Verification items for the finished model (mm, model axes). A direction names the side the tool comes from. Coordinates: 2 decimals unless noted, no trailing zeros. Order: outer loops, then holes, each group sorted by start corner. A loop starts at its lowest first (then second) coordinate and runs counter-clockwise, first axis right, second up. Notation, with made-up numbers: (10, 19.5) -> (47, 19.5) arc R24 ccw to (47, 39.5) -> close; hole circle Ø9 at (-11.75, 36). An arc over 180 degrees is marked (long way). Use CSV: the item, a comma, the result in double quotes. Start each with the question number.
1) Sectioned sample at A-A on z = -16. Record the boundary of the cut face in (x, y), then the cut area to 3 significant figures.
2) Go/stop test with flat-tipped pins: pin 1 (5 mm diameter, centred on x = 16, y = 8.5, fed in from -Z); pin 2 (5 mm diameter, centred on x = 5, z = -25, fed in from -Y); pin 3 (1.5 mm diameter, centred on y = 2, z = -17, fed in from +X); pin 4 (1 mm diameter, centred on x = 24, y = 8, fed in from +Z). Record where each tip stops, or that it passes through.
3) Sectioned sample at D-D on z = 0. Record the boundary of the cut face in (x, y).
4) Scan lines: line 1 along X through (y, z) = (2, -25); line 2 along Y through (x, z) = (0, -34); line 3 along X through (y, z) = (2, -26.5). Record each from-to range of solid material in increasing order.
5) Sectioned sample at C-C on x = 24.5. Record the boundary of the cut face in (y, z).
6) Tool access check on faces 4 (the cylindrical face through (4, 7.9, -53.7)), 5 (the flat face through (1.478, 7.93, -33.488)), 6 (the flat face through (12.5, 1, -16)). Record the directions out of +Z, -Z, +X, -X, +Y, -Y that give a thin tool (end or side, any length) a straight path to the whole face; none if there is none.
7) Release check for a two-part mould opening along Z. For faces 1 (the cylindrical face through (-7.186, 14.479, -39.317)), 2 (the cylindrical face through (12.186, 1.521, -5.276)), 3 (the flat face through (19.036, 7.888, -38.273)) record: released by +Z, released by -Z, zero draft, split by the parting line, or undercut.
8) Sectioned sample at B-B on y = 10.5. Record the boundary of the cut face in (x, z), then the cut area to 3 significant figures.
from build123d import *

# Parameters (mm, degrees)
SKETCH1_R           = 2
BOSS_EXTRUDE1_DEPTH = 3
FILLET1_R           = 10
BOSS_EXTRUDE2_DEPTH = 10
BOSS_EXTRUDE3_START = 10
SKETCH2_3_R         = 2
BOSS_EXTRUDE3_DEPTH = 3
CUT_EXTRUDE1_DEPTH  = 74.447466489


with BuildPart() as part:
    # Sketch1 → Boss-Extrude1 (new body)
    with BuildSketch(Plane(origin=(0, 0, 0), x_dir=(1, 0, 0), z_dir=(0, 1, 0))):
        Polygon((1.560538705, -15), (12.5, 5.232110419), (12.5, 31.328870119), (28.35, 39.898933149), (28.35, 66.496675358), (20.756215513, 66.496675358), (1.560538705, 56.117611626), (-7.5, 39.360495841), (-7.5, -15), align=None)
        with Locations(Location((0, 0, 0), (0, 0, 270))):
            Circle(SKETCH1_R, mode=Mode.SUBTRACT)
        with Locations(Location((5, 25, 0), (0, 0, 270))):
            Circle(SKETCH1_R, mode=Mode.SUBTRACT)
    extrude(amount=BOSS_EXTRUDE1_DEPTH)

    # Fillet1
    fillet1_edges = [part.edges().sort_by_distance(p)[0] for p in [
        (-7.5, 1.5, -39.360495841),
        (1.560538705, 1.5, -56.117611626),
        (20.756215513, 1.5, -66.496675358),
        (28.35, 1.5, -39.898933149),
        (12.5, 1.5, -31.328870119),
        (12.5, 1.5, -5.232110419),
        (1.560538705, 1.5, 15),
    ]]
    fillet(fillet1_edges, radius=FILLET1_R)

    # Sketch2 → Boss-Extrude2 (add)
    with BuildSketch(Plane(origin=(0, 3, 0), x_dir=(1, 0, 0), z_dir=(0, 1, 0))):
        with BuildLine():
            Line((-0.212131961, 34.733789396), (3.216589734, 32.20755665))
            ThreePointArc((3.216589734, 32.20755665), (9.62795757, 30.269843196), (15.824142619, 32.813003004))
            ThreePointArc((15.824142619, 32.813003004), (16.744165524, 33.545104209), (17.743757909, 34.164159444))
            Line((17.743757909, 34.164159444), (23.106242091, 37.063643824))
            ThreePointArc((23.106242091, 37.063643824), (26.939598969, 40.739700904), (28.35, 45.860129553))
            Line((28.35, 45.860129553), (28.35, 66.496675358))
            Line((28.35, 66.496675358), (23.286604522, 66.496675358))
            ThreePointArc((23.286604522, 66.496675358), (20.833530664, 66.191128856), (18.530362432, 65.293161086))
            Line((18.530362432, 65.293161086), (4.182884994, 57.535508975))
            ThreePointArc((4.182884994, 57.535508975), (1.868059273, 55.810091058), (0.142641356, 53.495265337))
            Line((0.142641356, 53.495265337), (-3.076922186, 47.54080713))
            ThreePointArc((-3.076922186, 47.54080713), (-4.039266122, 40.601621249), (-0.212131961, 34.733789396))
        make_face()
        with BuildLine():
            Line((1.56737669, 37.149022089), (4.996098385, 34.622789343))
            ThreePointArc((4.996098385, 34.622789343), (9.48405587, 33.266389925), (13.821385404, 35.046601791))
            ThreePointArc((13.821385404, 35.046601791), (15.017415181, 35.998333357), (16.316885282, 36.803105162))
            Line((16.316885282, 36.803105162), (21.679369463, 39.702589543))
            ThreePointArc((21.679369463, 39.702589543), (24.362719279, 42.275829499), (25.35, 45.860129553))
            Line((25.35, 45.860129553), (25.35, 63.496675358))
            Line((25.35, 63.496675358), (23.286604522, 63.496675358))
            ThreePointArc((23.286604522, 63.496675358), (21.569452821, 63.282792807), (19.957235059, 62.654215368))
            Line((19.957235059, 62.654215368), (5.609757621, 54.896563256))
            ThreePointArc((5.609757621, 54.896563256), (3.989379616, 53.688770715), (2.781587075, 52.06839271))
            Line((2.781587075, 52.06839271), (-0.437976468, 46.113934502))
            ThreePointArc((-0.437976468, 46.113934502), (-1.111617222, 41.256504386), (1.56737669, 37.149022089))
        make_face(mode=Mode.SUBTRACT)
    extrude(amount=BOSS_EXTRUDE2_DEPTH)

    # Sketch2<3> → Boss-Extrude3 (add)
    with BuildSketch(Plane(origin=(0, 3, 0), x_dir=(1, 0, 0), z_dir=(0, 1, 0)).offset(BOSS_EXTRUDE3_START)):
        with BuildLine():
            ThreePointArc((-3.076922186, 47.54080713), (-4.039266122, 40.601621249), (-0.212131961, 34.733789396))
            Line((-0.212131961, 34.733789396), (3.216589734, 32.20755665))
            ThreePointArc((3.216589734, 32.20755665), (9.62795757, 30.269843196), (15.824142619, 32.813003004))
            ThreePointArc((15.824142619, 32.813003004), (16.744165524, 33.545104209), (17.743757909, 34.164159444))
            Line((17.743757909, 34.164159444), (23.106242091, 37.063643824))
            ThreePointArc((23.106242091, 37.063643824), (26.939598969, 40.739700904), (28.35, 45.860129553))
            Line((28.35, 45.860129553), (28.35, 66.496675358))
            Line((28.35, 66.496675358), (23.286604522, 66.496675358))
            ThreePointArc((23.286604522, 66.496675358), (20.833530664, 66.191128856), (18.530362432, 65.293161086))
            Line((18.530362432, 65.293161086), (4.182884994, 57.535508975))
            ThreePointArc((4.182884994, 57.535508975), (1.868059273, 55.810091058), (0.142641356, 53.495265337))
            Line((0.142641356, 53.495265337), (-3.076922186, 47.54080713))
        make_face()
        with BuildLine():
            Line((4.996098385, 34.622789343), (1.56737669, 37.149022089))
            ThreePointArc((1.56737669, 37.149022089), (-1.111617222, 41.256504386), (-0.437976468, 46.113934502))
            Line((-0.437976468, 46.113934502), (2.781587075, 52.06839271))
            ThreePointArc((2.781587075, 52.06839271), (3.989379616, 53.688770715), (5.609757621, 54.896563256))
            Line((5.609757621, 54.896563256), (19.957235059, 62.654215368))
            ThreePointArc((19.957235059, 62.654215368), (21.569452821, 63.282792807), (23.286604522, 63.496675358))
            Line((23.286604522, 63.496675358), (25.35, 63.496675358))
            Line((25.35, 63.496675358), (25.35, 45.860129553))
            ThreePointArc((25.35, 45.860129553), (24.362719279, 42.275829499), (21.679369463, 39.702589543))
            Line((21.679369463, 39.702589543), (16.316885282, 36.803105162))
            ThreePointArc((16.316885282, 36.803105162), (15.017415181, 35.998333357), (13.821385404, 35.046601791))
            ThreePointArc((13.821385404, 35.046601791), (9.48405587, 33.266389925), (4.996098385, 34.622789343))
        make_face(mode=Mode.SUBTRACT)
        with BuildLine():
            Line((3.216589734, 32.20755665), (-0.212131961, 34.733789396))
            ThreePointArc((-0.212131961, 34.733789396), (-4.039266122, 40.601621249), (-3.076922186, 47.54080713))
            Line((-3.076922186, 47.54080713), (-6.296485729, 41.586348922))
            ThreePointArc((-6.296485729, 41.586348922), (-7.194453499, 39.28318069), (-7.5, 36.830106832))
            Line((-7.5, 36.830106832), (-7.5, -15))
            Line((-7.5, -15), (-4.400657699, -15))
            ThreePointArc((-4.400657699, -15), (0.71977095, -13.589598969), (4.39582803, -9.756242091))
            Line((4.39582803, -9.756242091), (11.296485729, 3.006257338))
            ThreePointArc((11.296485729, 3.006257338), (12.194453499, 5.30942557), (12.5, 7.762499429))
            Line((12.5, 7.762499429), (12.5, 25.367673715))
            ThreePointArc((12.5, 25.367673715), (13.368774074, 29.444524594), (15.824142619, 32.813003004))
            ThreePointArc((15.824142619, 32.813003004), (9.62795757, 30.269843196), (3.216589734, 32.20755665))
        make_face()
        with Locations(Location((0, 0, 0), (0, 0, 270))):
            Circle(SKETCH2_3_R, mode=Mode.SUBTRACT)
        with Locations(Location((5, 25, 0), (0, 0, 270))):
            Circle(SKETCH2_3_R, mode=Mode.SUBTRACT)
    extrude(amount=BOSS_EXTRUDE3_DEPTH)

    # Sketch4 → Cut-Extrude1 (cut, through all)
    with BuildSketch(Plane(origin=(0, 3, 0), x_dir=(1, 0, 0), z_dir=(0, 1, 0))):
        with BuildLine():
            Line((19.957235059, 62.654215368), (5.609757621, 54.896563256))
            ThreePointArc((5.609757621, 54.896563256), (3.989379616, 53.688770715), (2.781587075, 52.06839271))
            Line((2.781587075, 52.06839271), (-0.437976468, 46.113934502))
            ThreePointArc((-0.437976468, 46.113934502), (-1.111617222, 41.256504386), (1.56737669, 37.149022089))
            Line((1.56737669, 37.149022089), (4.996098385, 34.622789343))
            ThreePointArc((4.996098385, 34.622789343), (9.48405587, 33.266389925), (13.821385404, 35.046601791))
            ThreePointArc((13.821385404, 35.046601791), (15.017415181, 35.998333357), (16.316885282, 36.803105162))
            Line((16.316885282, 36.803105162), (21.679369463, 39.702589543))
            ThreePointArc((21.679369463, 39.702589543), (24.362719279, 42.275829499), (25.35, 45.860129553))
            Line((25.35, 45.860129553), (25.35, 63.496675358))
            Line((25.35, 63.496675358), (23.286604522, 63.496675358))
            ThreePointArc((23.286604522, 63.496675358), (21.569452821, 63.282792807), (19.957235059, 62.654215368))
        make_face()
    extrude(amount=-CUT_EXTRUDE1_DEPTH, mode=Mode.SUBTRACT)


solid = part.part
Answers follow:
1,outline,"(-7.5, 0) -> (12.5, 0) -> (12.5, 3) -> (-7.5, 3) -> close; (-7.5, 13) -> (12.5, 13) -> (12.5, 16) -> (-7.5, 16) -> close"
1,area,"120 mm²"
2,pin 1,"stops at z = -65.28"
2,pin 2,"stops at y = 0"
2,pin 3,"stops at x = 12.5"
2,pin 4,"stops at z = -37.29"
3,outline,"(-7.5, 0) -> (-2, 0) -> (-2, 3) -> (-7.5, 3) -> close; (-7.5, 13) -> (-2, 13) -> (-2, 16) -> (-7.5, 16) -> close; (2, 0) -> (9.67, 0) -> (9.67, 3) -> (2, 3) -> close; (2, 13) -> (9.67, 13) -> (9.67, 16) -> (2, 16) -> close"
4,line 1,"x = -7.5 to 3, 7 to 12.5"
4,line 2,"y = 0 to 3, 13 to 16"
4,line 3,"x = -7.5 to 3.68, 6.32 to 12.56"
5,outline,"(0, -66.5) -> (16, -66.5) -> (16, -63.5) -> (0, -63.5) -> close; (0, -42.52) -> (16, -42.52) -> (16, -37.97) -> (0, -37.97) -> close"
6,face 4,"+Y, -Y"
6,face 5,"+Z, -X"
6,face 6,"+Z, +X, +Y, -Y"
7,face 1,"released by -Z"
7,face 2,"released by +Z"
7,face 3,"undercut"
8,outline,"(-3.08, -47.54) -> (0.14, -53.5) arc R10 ccw to (4.18, -57.54) -> (18.53, -65.29) arc R10 ccw to (23.29, -66.5) -> (28.35, -66.5) -> (28.35, -45.86) arc R10 ccw to (23.11, -37.06) -> (17.74, -34.16) arc R10 cw to (15.82, -32.81) arc R10 ccw to (3.22, -32.21) -> (-0.21, -34.73) arc R10 ccw to start; hole (-0.44, -46.11) -> (2.78, -52.07) arc R7 ccw to (5.61, -54.9) -> (19.96, -62.65) arc R7 ccw to (23.29, -63.5) -> (25.35, -63.5) -> (25.35, -45.86) arc R7 ccw to (21.68, -39.7) -> (16.32, -36.8) arc R13 cw to (13.82, -35.05) arc R7 ccw to (5, -34.62) -> (1.57, -37.15) arc R7 ccw to start"
8,area,"303 mm²"
